Build history of the part. All positions in model axes, mm. Coordinates: 2 decimals unless noted, no trailing zeros. Loops run counter-clockwise (first coordinate to the right, second up) from the corner with the lowest first, then second, coordinate; pieces in that order, holes last. Notation, with made-up numbers: M 53.25,68 L 108.25,68 A16 cw 108.25,95 Z; hole C 64.5,-5 d10. An arc over 180 degrees is marked long. Write each question's results on one line, items separated by ' | '. Start each with the question number.
Autodesk Inventor part; units mm, degrees
ref_plane "YZ Plane" through (0, 0, 0) normal (1, 0, 0) x (0, 1, 0)
ref_plane "XZ Plane" through (0, 0, 0) normal (0, 1, 0) x (-1, 0, 0)
ref_plane "XY Plane" through (0, 0, 0) normal (0, 0, 1) x (1, 0, 0)
sketch "Sketch1" plane through (0, 0, 0) normal (0, 0, 1) x (1, 0, 0)
  line L0 (1, 4.5) -> (1, -4.5)
  line L1 (-1, -4.5) -> (-1, 4.5)
  arc A0 (1, 4.5) -> (-1, 4.5) centre (0, 4.5) ccw
  arc A1 (-1, -4.5) -> (1, -4.5) centre (0, -4.5) ccw
  line L2 (0, 5.5) -> (0, -5.5)
  point P0 (0, 0)
  point P1 (0, 0)
  dimension "d0" = 2
  dimension "d1" = 9
revolve "Revolution1" add sketch "Sketch1" angle 360 about axis through (0, 5.5, 0) along (0, -1, 0) contours L2 A1 L1 A0
sketch "Sketch3" plane through (0, 0, 0) normal (1, 0, 0) x (0, 1, 0)
  line L0 (8.5, 0.075) -> (4.5, 0.075)
  line L1 (4.5, 0.075) -> (4.5, -0.075)
  line L2 (4.5, -0.075) -> (8.5, -0.075)
  line L3 (8.5, -0.075) -> (8.5, 0.075)
  line L4 (0, 1.5086) -> (0, -1.8047) construction
  line L5 (6.5, -0.075) -> (7.5, -1.8071)
  line L6 (6.5, -0.075) -> (8.5, -0.075) construction
  line L7 (7.5, -1.8071) -> (7.6299, -1.7321)
  line L8 (7.6299, -1.7321) -> (6.5866, 0.075)
  line L9 (-8.5, 0.075) -> (-4.5, 0.075)
  line L10 (-4.5, 0.075) -> (-4.5, -0.075)
  line L11 (-4.5, -0.075) -> (-8.5, -0.075)
  line L12 (-8.5, -0.075) -> (-8.5, 0.075)
  line L13 (-6.5, -0.075) -> (-7.5, -1.8071)
  line L14 (-6.5, -0.075) -> (-8.5, -0.075) construction
  line L15 (-7.5, -1.8071) -> (-7.6299, -1.7321)
  line L16 (-7.6299, -1.7321) -> (-6.5866, 0.075)
  point P0 (0, 0)
  dimension "d7" = 4
  dimension "d8" = 0.15
  dimension "d11" = 2
  dimension "d12" = 60
  dimension "d13" = 0.15
  dimension "d14" = 4.5
extrude "Extrusion2" add sketch "Sketch3" along normal mid plane 0.8 contours L8 L2 L1 L0 | L8 L7 L5 L2 | L9 L10 L11 L16 | L11 L13 L15 L16
properties part number "LED Filament"
1. Mould opens along Y. For faces 1 (the flat face through (-0.006, 6.993, -0.929)), 2 (the flat face through (-0.006, 7.116, -0.841)), 3 (the flat face through (-0.006, -7.116, -0.841)) say: +Y half, -Y half, draft (parallel to the pull), parting line (faces both ways), or undercut.
2. Band-saw the part on A-A, the plane z = -1.3. List the corners of the cut face in (x, y), plus the area to 3 significant figures.
3. Pin check, flat tips, straight feed: pin 1 (0.6 mm diameter, centred on x = 0, y = 6, fed in from -Z) (3 decimals); pin 2 (0.9 mm diameter, centred on y = 7, z = -1.5, fed in from -X); pin 3 (1 mm diameter, centred on x = 0.5, z = 0, fed in from +Y). Stop position of each tip, or through.
4. Wall check: line 1 along Y through (x, z) = (0.2, -0.6); line 2 along Y through (x, z) = (-0.35, -0.8); line 3 along Z through (x, y) = (0, 2.5). Give the ranges that are in metal, low to high.
5. Band-saw the part on D-D, the plane y = -4. List the corners of the cut face in (x, z), plus the area to 3 significant figures.
6. Band-saw the part on B-B, the plane x = 0. List the corners of the cut face in (y, z) (3 decimals).
7. Band-saw the part on C-C, the plane z = -0.5. List the corners of the cut face in (x, y), plus the area to 3 significant figures.
Checked values:
1) face 1: undercut | face 2: +Y half | face 3: -Y half
2) outline: M -0.4,-7.38 L 0.4,-7.38 L 0.4,-7.21 L -0.4,-7.21 Z; M -0.4,7.21 L 0.4,7.21 L 0.4,7.38 L -0.4,7.38 Z | area: 0.277 mm²
3) pin 1: z = -0.075 | pin 2: x = -0.4 | pin 3: y = 6.91
4) line 1: -6.98 to -6.8, -5.27 to 5.27, 6.8 to 6.98 | line 2: -7.09 to -6.92, -4.99 to 4.99, 6.92 to 7.09 | line 3: -1 to 1
5) outline: C 0,0 d2 | area: 3.14 mm²
6) outline: M -7.63,-1.732 L -7.5,-1.807 L -6.5,-0.075 L -5.497,-0.075 A1 ccw -4.5,-1 L 4.5,-1 A1 ccw 5.497,-0.075 L 6.5,-0.075 L 7.5,-1.807 L 7.63,-1.732 L 6.587,0.075 L 5.497,0.075 A1 ccw 4.5,1 L -4.5,1 A1 ccw -5.497,0.075 L -6.587,0.075 Z
7) outline: M -0.87,-4.5 A0.87 ccw 0.87,-4.5 L 0.87,4.5 A0.87 ccw -0.87,4.5 Z; M -0.4,-6.92 L 0.4,-6.92 L 0.4,-6.75 L -0.4,-6.75 Z; M -0.4,6.75 L 0.4,6.75 L 0.4,6.92 L -0.4,6.92 Z | area: 18.2 mm²
